from build123d import *

# Parameters (mm, degrees)
F0_W      = 68.58
F0_H      = 68.58
F1_DEPTH  = 68.58
F2_R      = 28.575
F3_DEPTH  = 10.795
F4_R      = 28.575
F5_DEPTH  = 10.795
F6_R      = 28.575
F7_DEPTH  = 10.795
F8_R      = 28.575
F9_DEPTH  = 10.795
F10_R     = 28.575
F11_DEPTH = 10.795
F12_R     = 28.575
F13_DEPTH = 10.795
F14_R     = 19.05
F15_DEPTH = 8.89
F16_R     = 19.05
F17_DEPTH = 8.89
F18_R     = 19.05
F19_DEPTH = 8.89
F20_R     = 19.05
F21_DEPTH = 8.89
F22_R     = 19.05
F23_DEPTH = 8.89
F24_R     = 19.05
F25_DEPTH = 8.89
F26_R     = 11.1125
F27_DEPTH = 6.35
F28_R     = 11.1125
F29_DEPTH = 6.35
F30_R     = 11.1125
F31_DEPTH = 6.35
F32_R     = 11.1125
F33_DEPTH = 6.35
F34_R     = 11.1125
F35_DEPTH = 6.35
F36_R     = 11.1125
F37_DEPTH = 6.35


with BuildPart() as f1:
    # F0 (on Front) → F1 (new body)
    with BuildSketch(Plane.XZ):
        with Locations((10.824279, -2.404214)):
            Rectangle(F0_W, F0_H)
    extrude(amount=F1_DEPTH)

    # F2 (on face) → F3 (cut)
    with BuildSketch(Plane.XZ.offset(68.58)):
        with Locations((10.824279, -2.404214)):
            Circle(F2_R)
    extrude(amount=-F3_DEPTH, mode=Mode.SUBTRACT)

    # F4 (on face) → F5 (cut)
    with BuildSketch(Plane.YZ.offset(45.114279)):
        with Locations((-34.29, -2.404214)):
            Circle(F4_R)
    extrude(amount=-F5_DEPTH, mode=Mode.SUBTRACT)

    # F6 (on face) → F7 (cut)
    with BuildSketch(Plane(origin=(0, 0, 0), x_dir=(-1, 0, 0), z_dir=(0, 1, 0))):
        with Locations((-10.824279, -2.404214)):
            Circle(F6_R)
    extrude(amount=-F7_DEPTH, mode=Mode.SUBTRACT)

    # F8 (on face) → F9 (cut)
    with BuildSketch(Plane(origin=(-23.465721, 0, 0), x_dir=(0, -1, 0), z_dir=(-1, 0, 0))):
        with Locations((34.29, -2.404214)):
            Circle(F8_R)
    extrude(amount=-F9_DEPTH, mode=Mode.SUBTRACT)

    # F10 (on face) → F11 (cut)
    with BuildSketch(Plane.XY.offset(31.885786)):
        with Locations((10.824279, -34.29)):
            Circle(F10_R)
    extrude(amount=-F11_DEPTH, mode=Mode.SUBTRACT)

    # F12 (on face) → F13 (cut)
    with BuildSketch(Plane(origin=(0, 0, -36.694214), x_dir=(1, 0, 0), z_dir=(0, 0, -1))):
        with Locations((10.824279, 34.29)):
            Circle(F12_R)
    extrude(amount=-F13_DEPTH, mode=Mode.SUBTRACT)

    # F14 (on face) → F15 (cut)
    with BuildSketch(Plane.XZ.offset(57.785)):
        with Locations((10.824279, -2.404214)):
            Circle(F14_R)
    extrude(amount=-F15_DEPTH, mode=Mode.SUBTRACT)

    # F16 (on face) → F17 (cut)
    with BuildSketch(Plane.YZ.offset(34.319279)):
        with Locations((-34.29, -2.404214)):
            Circle(F16_R)
    extrude(amount=-F17_DEPTH, mode=Mode.SUBTRACT)

    # F18 (on face) → F19 (cut)
    with BuildSketch(Plane(origin=(0, -10.795, 0), x_dir=(-1, 0, 0), z_dir=(0, 1, 0))):
        with Locations((-10.824279, -2.404214)):
            Circle(F18_R)
    extrude(amount=-F19_DEPTH, mode=Mode.SUBTRACT)

    # F20 (on face) → F21 (cut)
    with BuildSketch(Plane(origin=(-12.670721, 0, 0), x_dir=(0, -1, 0), z_dir=(-1, 0, 0))):
        with Locations((34.29, -2.404214)):
            Circle(F20_R)
    extrude(amount=-F21_DEPTH, mode=Mode.SUBTRACT)

    # F22 (on face) → F23 (cut)
    with BuildSketch(Plane.XY.offset(21.090786)):
        with Locations((10.824279, -34.29)):
            Circle(F22_R)
    extrude(amount=-F23_DEPTH, mode=Mode.SUBTRACT)

    # F24 (on face) → F25 (cut)
    with BuildSketch(Plane(origin=(0, 0, -25.899214), x_dir=(1, 0, 0), z_dir=(0, 0, -1))):
        with Locations((10.824279, 34.29)):
            Circle(F24_R)
    extrude(amount=-F25_DEPTH, mode=Mode.SUBTRACT)

    # F26 (on face) → F27 (cut)
    with BuildSketch(Plane.YZ.offset(25.429279)):
        with Locations((-34.29, -2.404214)):
            Circle(F26_R)
    extrude(amount=-F27_DEPTH, mode=Mode.SUBTRACT)

    # F28 (on face) → F29 (cut)
    with BuildSketch(Plane.XY.offset(12.200786)):
        with Locations((10.824279, -34.29)):
            Circle(F28_R)
    extrude(amount=-F29_DEPTH, mode=Mode.SUBTRACT)

    # F30 (on face) → F31 (cut)
    with BuildSketch(Plane.XZ.offset(48.895)):
        with Locations((10.824279, -2.404214)):
            Circle(F30_R)
    extrude(amount=-F31_DEPTH, mode=Mode.SUBTRACT)

    # F32 (on face) → F33 (cut)
    with BuildSketch(Plane(origin=(0, -19.685, 0), x_dir=(-1, 0, 0), z_dir=(0, 1, 0))):
        with Locations((-10.824279, -2.404214)):
            Circle(F32_R)
    extrude(amount=-F33_DEPTH, mode=Mode.SUBTRACT)

    # F34 (on face) → F35 (cut)
    with BuildSketch(Plane(origin=(0, 0, -17.009214), x_dir=(1, 0, 0), z_dir=(0, 0, -1))):
        with Locations((10.824279, 34.29)):
            Circle(F34_R)
    extrude(amount=-F35_DEPTH, mode=Mode.SUBTRACT)

    # F36 (on face) → F37 (cut)
    with BuildSketch(Plane(origin=(-3.780721, 0, 0), x_dir=(0, -1, 0), z_dir=(-1, 0, 0))):
        with Locations((34.29, -2.404214)):
            Circle(F36_R)
    extrude(amount=-F37_DEPTH, mode=Mode.SUBTRACT)


solid = f1.part
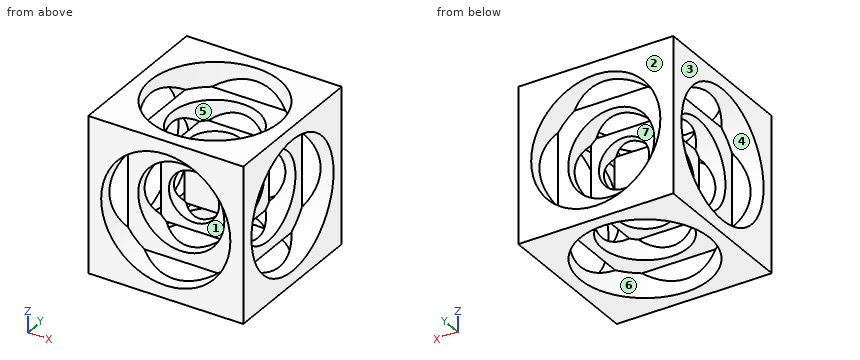
Could you check a few things on this model? Use its own coordinates, in mm. Face numbers are marked on the shaded views. A direction names the side the tool comes from. Give positions to 0.01 mm unless a question says otherwise; leave off trailing zeros. Order: outer loops, then holes, each group sorted by start corner. A loop starts at its lowest first (then second) coordinate and runs counter-clockwise, first axis right, second up.
Item 1: I need wall thicknesses on line 1 (Y direction, x = 28, z = 18.5) (3 decimals); line 2 (Y direction, x = 34, z = -33); line 3 (Z direction, x = 10, y = -29). Which ranges of each line are inside material? Lowest first, please.
Item 2: I'm going to push flat-ended pins straight in: pin 1 (8.5 mm diameter, centred on x = 8, z = 0, fed in from +Y) (3 decimals); pin 2 (14.5 mm diameter, centred on y = -31.5, z = 0, fed in from -X); pin 3 (14 mm diameter, centred on x = 11, z = -11.5, fed in from +Y) (3 decimals). Where does each tip first touch, or does it pass through?
Item 3: If we section it at A-A, the plane y = -34.29: Count the separate pieces of the cut face and the enclosed holes in it, plus the area to 3 significant figures.
Item 4: For the marked faces 5, 6 and 7, which set-ups out of +Z, -Z, +X, -X, +Y, -Y let a thin tool reach every point of the face, with its end or its side?
Item 5: If we section it at B-B, the plane y = -60: Write out the boundary of the cut face in (x, z) (3 decimals).
Item 6: If we mould it in two halves opening along Y, with no side actions, what happens to the marked faces 1, 2, 3 and 4? For each: pulls with the +Y half, pulls with the -Y half, needs draft (parallel to the pull), parting line crosses it, or undercut.
Values:
1. line 1: y = -57.785 to -42.53, -26.05 to -10.795
1. line 2: y = -68.58 to -51.01, -17.57 to 0
1. line 3: z = -10.66 to 5.85
2. pin 1: stops at y = -26.035
2. pin 2: stops at x = 2.57
2. pin 3: stops at y = -19.685
3. separate pieces: 13
3. enclosed holes: 0
3. area: 531 mm2
4. face 5: +Z
4. face 6: -Z
4. face 7: +Y
5. outline: (-23.466, -36.694) - (-1.647, -36.694) - (-1.647, -28.114) arc R28.575 cw to (-14.886, -14.875) - (-23.466, -14.875) - close; (-23.466, 10.067) - (-14.886, 10.067) arc R28.575 cw to (-1.647, 23.306) - (-1.647, 31.886) - (-23.466, 31.886) - close; (23.295, -36.694) - (45.114, -36.694) - (45.114, -14.875) - (36.534, -14.875) arc R28.575 cw to (23.295, -28.114) - close; (23.295, 23.306) arc R28.575 cw to (36.534, 10.067) - (45.114, 10.067) - (45.114, 31.886) - (23.295, 31.886) - close
6. face 1: pulls with the -Y half
6. face 2: pulls with the +Y half
6. face 3: needs draft
6. face 4: undercut
